For this review, take the finished solid that the model builds, in its own axes (mm). Face numbers are marked on the shaded views. A direction names the side the tool comes from. Coordinates: 2 decimals unless noted, no trailing zeros. Loops run counter-clockwise (first coordinate to the right, second up) from the corner with the lowest first, then second, coordinate; pieces in that order, holes last. Notation, with made-up numbers: M 69,85.5 L 86,85.5 A22 ccw 86,105.5 Z; hole C -28.75,53 d7. An arc over 180 degrees is marked long. Write item = value, one per line.
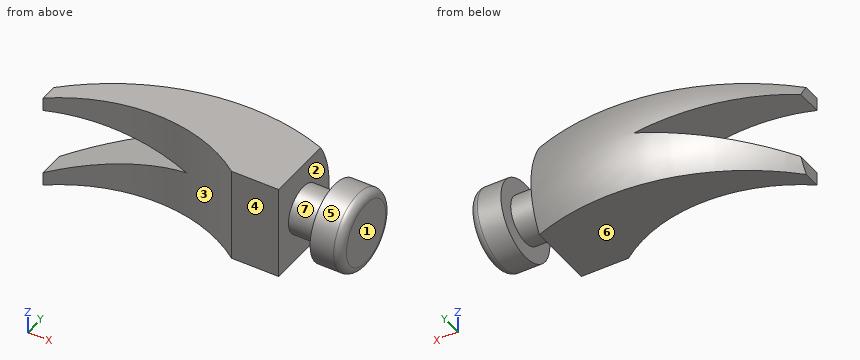
from build123d import *

# Parameters (mm, degrees)
BOSS_EXTRUDE1_DEPTH     = 30
SKETCH3_OUTSIDE_W       = 103.618
SKETCH3_OUTSIDE_H       = 103.618
SKETCH3_OUTSIDE_R       = 25
CUT_EXTRUDE1_DEPTH      = 40
CUT_EXTRUDE2_START      = -20
SKETCH4_OUTSIDE_W       = 103.618
SKETCH4_OUTSIDE_H       = 103.618
SKETCH4_OUTSIDE_R       = 15
CUT_EXTRUDE2_DEPTH      = 20
FILLET1_R               = 5
CUT_EXTRUDE3_REACH      = 148.287
CUT_EXTRUDE3_END_RADIUS = 150


with BuildPart() as part:
    # Sketch2 → Boss-Extrude1 (new, symmetric)
    with BuildSketch(Plane.XY):
        with BuildLine():
            Line((-60, 80), (-60, 101.803398875))
            ThreePointArc((-60, 101.803398875), (10.943058496, 137.158737934), (90, 131.421356237))
            Line((90, 131.421356237), (90, 120))
            Line((90, 120), (110, 120))
            Line((110, 120), (110, 130))
            Line((110, 130), (130, 130))
            Line((130, 130), (130, 80))
            Line((130, 80), (110, 80))
            Line((110, 80), (110, 90))
            Line((110, 90), (90, 90))
            Line((90, 90), (90, 80))
            Line((90, 80), (60, 80))
            ThreePointArc((60, 80), (0, 100), (-60, 80))
        make_face()
    extrude(amount=BOSS_EXTRUDE1_DEPTH, both=True)

    # Sketch3 outside → Cut-Extrude1 (cut)
    with BuildSketch(Plane(origin=(130, 0, 0), x_dir=(0, 0, -1), z_dir=(1, 0, 0))):
        with Locations((0, 110)):
            Rectangle(SKETCH3_OUTSIDE_W, SKETCH3_OUTSIDE_H)
        with Locations((0, 105)):
            Circle(SKETCH3_OUTSIDE_R, mode=Mode.SUBTRACT)
    extrude(amount=-CUT_EXTRUDE1_DEPTH, mode=Mode.SUBTRACT)

    # Sketch4 outside → Cut-Extrude2 (cut)
    with BuildSketch(Plane(origin=(130, 0, 0), x_dir=(0, 0, -1), z_dir=(1, 0, 0)).offset(CUT_EXTRUDE2_START)):
        with Locations((0, 110)):
            Rectangle(SKETCH4_OUTSIDE_W, SKETCH4_OUTSIDE_H)
        with Locations((0, 105)):
            Circle(SKETCH4_OUTSIDE_R, mode=Mode.SUBTRACT)
    extrude(amount=-CUT_EXTRUDE2_DEPTH, mode=Mode.SUBTRACT)

    # Fillet1
    fillet1_edges = [part.edges().sort_by_distance(p)[0] for p in [
        (130, 105, 25),
    ]]
    fillet(fillet1_edges, radius=FILLET1_R)

    # Cut-Extrude3: up to this cylinder (the profile starts inside it)
    cut_extrude3_end = Plane(origin=(40, -10, 0), z_dir=(0, 0, -1)) * Cylinder(CUT_EXTRUDE3_END_RADIUS, 597.574, mode=Mode.PRIVATE)
    # Sketch5 → Cut-Extrude3 (cut, up to the surface)
    with BuildSketch(Plane.XZ.offset(-80), mode=Mode.PRIVATE) as cut_extrude3_sk1:
        Polygon((20, 0), (-60, 21.435935394), (-60, -21.435935394), align=None)
    cut_extrude3_tool1 = extrude(cut_extrude3_sk1.sketch, amount=-CUT_EXTRUDE3_REACH, mode=Mode.PRIVATE) & cut_extrude3_end
    add(cut_extrude3_tool1.solids().sort_by_distance((-33.333333, 80, 0))[0], mode=Mode.SUBTRACT)

    # SurfaceCut4: cut with a surface, the side it looks to stays
    # Surface-Sweep1: a surface, the sketch's curves swept along a path
    with BuildLine(Plane(origin=(40, 0, 0), x_dir=(0, 0, -1), z_dir=(1, 0, 0)), mode=Mode.PRIVATE) as surface_sweep1_1_profile:
        Line((0, 20), (0, 80))
        Line((0, 80), (60, 80))
        ThreePointArc((60, 80), (-42.426406871, 122.426406871), (0, 20))
    with BuildLine(Plane.XY, mode=Mode.PRIVATE) as surface_sweep1_1_along:
        ThreePointArc((104.347571597, 125.49682664), (-0.649478186, 134.387049015), (-85.586612969, 72.024402728))
    surface_sweep1_1 = Shell.sweep(surface_sweep1_1_profile.wire(), surface_sweep1_1_along.wire())
    split(bisect_by=surface_sweep1_1, keep=Keep.TOP)


solid = part.part
Q1. Draft analysis for pull direction X (two halves, no side actions). For the marked faces 1, 2, 3 and 4, state which applies: +X half, -X half, draft (parallel to the pull), parting line (faces both ways), or undercut.
Solved:
face_1 = +X half
face_2 = undercut
face_3 = undercut
face_4 = draft
Q2. For line 1 along Y through (x, z) = (96.5, 0); line 2 along X through (y, z) = (83.5, -5) (3 decimals); line 3 along X through (y, z) = (88, 4.5), list the stretches that pass through material, from the lowest coordinate up.
Solved:
line_1 = 90 to 120
line_2 = 55.025 to 90, 110 to 129.55
line_3 = 47.5 to 90, 110 to 130
Q3. Machinability: for the marked faces 5, 6 and 7, which of the approach directions +Z, -Z, +X, -X, +Y, -Y give a long, thin tool a straight path to every point of the face, cutting with its end or side? Answer none if there is none.
Solved:
face_5 = +X
face_6 = -Z, +X, -X, +Y, -Y
face_7 = none
Q4. For pin 1 Ø10 at (x, y) = (111, 96) entering from -Z; pin 2 Ø1.5 at (x, z) = (16, 24) entering from +Y, all flat-tipped, find the tip position at first contact; note any pin that passes through.
Solved:
pin_1 = -24.68
pin_2 = 133.34
Q5. Add section A-A (x = 114.5). Write out the cut boundary in (y, z).
Solved:
outline = C 105,0 d50
